Can you work these out from the drawing? Everything is in mm from the part's minimum corner. Give positions to 0.01 mm unless a question says otherwise; leave off trailing zeros. Loops run counter-clockwise (first coordinate to the right, second up) from the corner with the lowest first, then second, coordinate; pieces in that order, holes last. Notation, with made-up numbers: M -5.5,69 L 37.5,69 A24 cw 37.5,101 Z; hole C 16.25,1.25 d4. An arc over 180 degrees is marked long. Use CSV: the item, a comma, the result in double quotes.
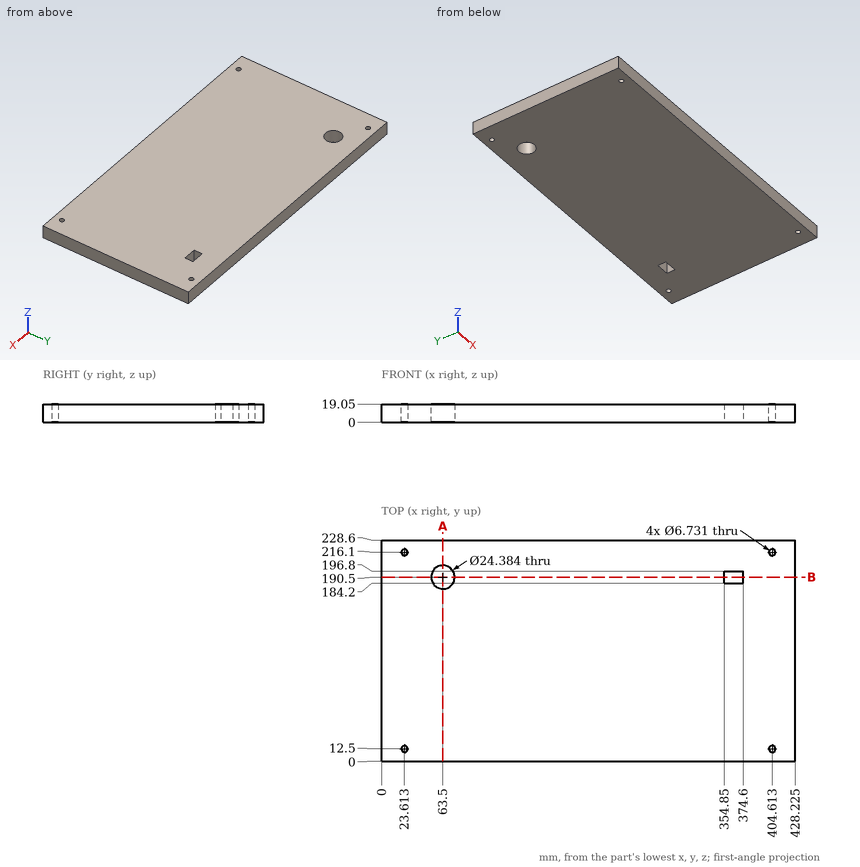
Q1. Please list where these lines run through material, in increasing order: L1, parallel to Y at x = 24, z = 16.75; L2, parallel to Y at x = 407.5, z = 16 (1 decimal); L3, parallel to Y at x = 63.5, z = 10. Write a range as from..to.
Model answer:
L1,"0..9.16, 15.84..212.76, 219.44..228.6"
L2,"0..10.8, 14.2..214.4, 217.8..228.6"
L3,"0..178.31, 202.69..228.6"
Q2. I want a section at A-A, the plane x = 63.5. Please give me the cut outline in (y, z), then the cut area to 3 significant figures.
Model answer:
outline,"M 0,0 L 178.31,0 L 178.31,19.05 L 0,19.05 Z; M 202.69,0 L 228.6,0 L 228.6,19.05 L 202.69,19.05 Z"
area,"3,890 mm2"
Q3. I want a section at B-B, the plane y = 190.5. State how many separate pieces and enclosed holes the cut face has, then the cut area to 3 significant figures.
Model answer:
separate pieces,"3"
enclosed holes,"0"
area,"7,320 mm2"
Q4. I'm going to push a flat-ended pin straight in: P1, Ø6, axis at x = 404.61, y = 216.1, coming from the +Z side. Where does the tip first touch, or does it pass through?
Model answer:
P1,"through"
